Source: CAD feature listing. Evaluate the final solid. Frame: model axes, mm. A direction names the side the tool comes from. Give positions to 0.01 mm unless a question says otherwise; leave off trailing zeros. Write each loop counter-clockwise with the first axis right and the second up, starting at its lowest first coordinate (ties: lowest second). Pieces come first, ordered by that corner, then holes. Notation, with made-up numbers: M -21.5,-26.75 L -2.5,-26.75 A7 cw -2.5,-22.75 Z; hole C 6.5,28 d9. An arc over 180 degrees is marked long. Use CSV: the item, a comma, the result in double quotes. Start each with the question number.
from build123d import *

# Parameters (mm, degrees)
SKETCH_1_W          = 42
SKETCH_1_H          = 78
EXTRUDE_1_DEPTH     = 17
FILLET_1_R          = 5
SKETCH_2_R          = 2.810395333
SKETCH_2_W          = 23.945669991
SKETCH_2_H          = 2.577112466
SKETCH_2_W_2        = 15.24791542
SKETCH_2_H_2        = 2.362353093
SKETCH_2_H_3        = 2.577112465
SKETCH_2_H_4        = 2.684492151
SKETCH_2_H_5        = 2.147593721
CUT_EXTRUDE_1_DEPTH = 1
SKETCH_3_R          = 1.971229003
EXTRUDE_2_DEPTH     = 3
FILLET_2_R          = 1


with BuildPart() as part:
    # Эскиз1 → Бобышка-Вытянуть1 (new body)
    with BuildSketch(Plane.XY):
        with Locations((4.449416517, -23.815978456)):
            Rectangle(SKETCH_1_W, SKETCH_1_H)
    extrude(amount=EXTRUDE_1_DEPTH)

    # Скругление1
    fillet_1_edges = [part.edges().sort_by_distance(p)[0] for p in [
        (25.449416517, -23.815978456, 17),
        (4.449416517, 15.184021544, 17),
        (-16.550583483, -23.815978456, 17),
        (4.449416517, -62.815978456, 17),
    ]]
    fillet(fillet_1_edges, radius=FILLET_1_R)

    # Эскиз2 → Вырез-Вытянуть1 (cut)
    with BuildSketch(Plane.XY.offset(17)):
        with Locations((12.341823442, -5.239292768)):
            Circle(SKETCH_2_R)
        with Locations((4.878935262, 3.136322744)):
            Rectangle(SKETCH_2_W, SKETCH_2_H)
        with Locations((0.530057976, -5.239292769)):
            Rectangle(SKETCH_2_W_2, SKETCH_2_H_2)
        with Locations((4.878935262, -12.863250478)):
            Rectangle(SKETCH_2_W, SKETCH_2_H_3)
        with Locations((4.878935262, -19.735550386)):
            Rectangle(SKETCH_2_W, SKETCH_2_H)
        with Locations((4.878935262, -26.446780765)):
            Rectangle(SKETCH_2_W, SKETCH_2_H_4)
        with Locations((4.878935262, -33.909668946)):
            Rectangle(SKETCH_2_W, SKETCH_2_H_5)
        with Locations((4.878935262, -40.996728225)):
            Rectangle(SKETCH_2_W, SKETCH_2_H)
        with Locations((4.878935262, -50.12400154)):
            Rectangle(SKETCH_2_W, SKETCH_2_H_3)
    extrude(amount=-CUT_EXTRUDE_1_DEPTH, mode=Mode.SUBTRACT)

    # Эскиз3 → Бобышка-Вытянуть2 (add)
    with BuildSketch(Plane.XY.offset(16)):
        with Locations((12.341823442, -5.239292768)):
            Circle(SKETCH_3_R)
    extrude(amount=EXTRUDE_2_DEPTH)

    # Скругление2
    fillet_2_edges = [part.edges().sort_by_distance(p)[0] for p in [
        (10.370594439, -5.239292768, 19),
    ]]
    fillet(fillet_2_edges, radius=FILLET_2_R)


solid = part.part
1. First-contact query: pin 1 (0.5 mm diameter, centred on y = -49.5, z = 16.5, fed in from +X); pin 2 (0.8 mm diameter, centred on x = 5.5, z = 16.5, fed in from -Y); pin 3 (0.8 mm diameter, centred on y = -20, z = 16.5, fed in from -X). Flat tips, straight axial feed; report the tip coordinate or a pass-through.
2. Section B-B on z = 14.5. Return loops of the section in (x, y), then the cut area to 3 significant figures.
3. Pull-direction query (Y, two-part tool) for faces 1 (the flat face through (5, -41, 16)), 2 (the flat face through (25.449, -24, 6)), 3 (the flat face through (4, -62.816, 6)); classes: released by +Y, released by -Y, zero draft, split by the parting line, or undercut.
4. Line query: probe 1 along Z at (x, y) = (14, -47.5); probe 2 along X at (y, z) = (-40, 12.25); probe 3 along Y at (x, z) = (0, 12.25). Output: solid intervals per line, ascending.
5. Access query for faces 4 (the flat face through (5, -26, 16)), 5 (the cylindrical face through (4.743, -61.39, 15.496)). Directions: +Z, -Z, +X, -X, +Y, -Y. A direction counts if a zero-diameter tool reaches every point of the face in a straight line with its end or side. Return the directions, or none.
6. Section A-A on y = -36. Return loops of the section in (x, z).
Resolved:
1,pin 1,"stops at x = 23.08"
1,pin 2,"stops at y = -60.68"
1,pin 3,"stops at x = -14.41"
2,outline,"M -15.88,-62.15 L 24.78,-62.15 L 24.78,14.51 L -15.88,14.51 Z"
2,area,"3,120 mm2"
3,face 1,"undercut"
3,face 2,"zero draft"
3,face 3,"released by -Y"
4,probe 1,"z = 0 to 17"
4,probe 2,"x = -16.54 to 25.44"
4,probe 3,"y = -62.81 to 15.18"
5,face 4,"+Z"
5,face 5,"+Z, +X, -X, -Y"
6,outline,"M -16.55,0 L 25.45,0 L 25.45,12 A5 ccw 20.45,17 L -11.55,17 A5 ccw -16.55,12 Z"
